The listing builds one solid part. Answer for the finished solid, in the listing's coordinates (mm). A direction names the side the tool comes from. Round coordinates to 2 decimals unless told otherwise and drop trailing zeros. Loops run counter-clockwise (first coordinate to the right, second up) from the corner with the lowest first, then second, coordinate; pieces in that order, holes last. Notation, with made-up numbers: (51, 19) -> (94, 19) arc R14 ccw to (94, 34) -> close; hole circle Ø5 at (-4, 55.5). An arc over 180 degrees is marked (long way). Write each question's results on one line, items separated by ' | '. Start each with the question number.
(1) For faces 5 (the face through (24.599, 16.868, -11.668)), 6 (the face through (22.67, 7.94, -7.07)), 7 (the face through (17.455, 12, -49)), 8 (the face through (18, 18.622, -43)), determine the directions among +Z, -Z, +X, -X, +Y, -Y from which every point of the face is accessible in a straight line to the end or side of a thin tool.
(2) The part is cut by section B-B (y = 4.5). Determine the outline of the cut face in (x, z).
(3) The part is cut by section C-C (x = 15). Determine the outline of the cut face in (y, z), plus the area to 3 significant figures.
(4) Straight lines are drawn through the part: probe 1 along Z at (x, y) = (11.75, 11.5); probe 2 along Y at (x, z) = (18.25, -6). For each, find the intervals that lie inside material, in ascending order.
(5) Determine the mould class of faces 1 (the face through (11.35, 18.05, -42.93)), 2 (the face through (18.144, 12.138, -10.497)), 3 (the face through (18, 0.622, -43)), 4 (the face through (19.226, 12.217, -5.07)) for opening direction Y: released by +Y, released by -Y, zero draft, split by the parting line, or undercut.
(6) The part is cut by section A-A (z = -45). Determine the outline of the cut face in (x, y), plus the area to 3 significant figures.
(7) The part is cut by section D-D (y = 7.5). Determine the outline of the cut face in (x, z).
(8) Flat-ended cylindrical pins translate along their axes: pin 1 (1.6 mm diameter, centred on y = 12, z = -48.5, fed in from +X); pin 2 (1.8 mm diameter, centred on x = 18.25, y = 12, fed in from +Z); pin 3 (3 mm diameter, centred on x = 18.5, z = -45.5, fed in from +Y); pin 4 (5 mm diameter, centred on x = 20, y = 15, fed in from +Z). Find the tip coordinate at first contact, or state that the pin passes through.
Autodesk Inventor part; units mm, degrees
ref_plane "YZ Plane" through (0, 0, 0) normal (1, 0, 0) x (0, 1, 0)
ref_plane "XZ Plane" through (0, 0, 0) normal (0, 1, 0) x (-1, 0, 0)
ref_plane "XY Plane" through (0, 0, 0) normal (0, 0, 1) x (1, 0, 0)
sketch "Sketch1" plane through (0, 0, 0) normal (0, 0, 1) x (1, 0, 0)
  arc A0 (10.5041, 10) -> (25.996, 10) centre (18.25, 12) ccw
  circle A1 centre (18.25, 12) radius 8
  point P0 (0, 0)
extrude "Extrusion1" add sketch "Sketch1" against normal blind 4.8
sketch "Sketch2" plane through (18.25, 12, -4.8) normal (0, 0, -1) x (-1, 0, 0)
  circle A0 centre (0, 0) radius 8
  circle A1 centre (0, 0) radius 6
  point P0 (18.25, -12)
  dimension "d2" = 12
extrude "Extrusion2" add sketch "Sketch2" along normal blind 4.6 contours A1
sketch "Sketch3" plane through (18.25, 12, -9.4) normal (0, 0, -1) x (-1, 0, 0)
  circle A0 centre (0, 0) radius 6
  circle A1 centre (0, 0) radius 8
  point P0 (18.25, -12)
extrude "Extrusion3" add sketch "Sketch3" along normal blind 4.6 contours A0 | A1
sketch "Sketch4" plane through (18.25, 12, -14) normal (0, 0, -1) x (-1, 0, 0)
  circle A0 centre (0, 0) radius 8
  circle A1 centre (0, 0) radius 5
  point P0 (18.25, -12)
  dimension "d7" = 10
extrude "Extrusion4" add sketch "Sketch4" along normal blind 24 contours A1
thread "Thread1"
sketch "Sketch5" plane through (18.25, 12, -38) normal (0, 0, -1) x (-1, 0, 0)
  line L0 (-5.5007, -11.3783) -> (5.4993, -11.3783)
  line L1 (7.4993, -9.3783) -> (7.4993, 4.6217)
  line L2 (5.4993, 6.6217) -> (-5.5007, 6.6217)
  line L3 (-7.5007, 4.6217) -> (-7.5007, -9.3783)
  line L4 (-7.5007, -11.3783) -> (7.4993, 6.6217) construction
  line L5 (7.4993, -11.3783) -> (-7.5007, 6.6217) construction
  arc A0 (7.4993, 4.6217) -> (5.4993, 6.6217) centre (5.4993, 4.6217) ccw
  arc A1 (-5.5007, 6.6217) -> (-7.5007, 4.6217) centre (-5.5007, 4.6217) ccw
  arc A2 (-7.5007, -9.3783) -> (-5.5007, -11.3783) centre (-5.5007, -9.3783) ccw
  arc A3 (5.4993, -11.3783) -> (7.4993, -9.3783) centre (5.4993, -9.3783) ccw
  point P0 (18.25, -12)
  point P1 (-0.0007, -2.3783)
  dimension "d12" = 15
  dimension "d13" = 18
  dimension "d14" = 2
extrude "Extrusion5" add sketch "Sketch5" along normal blind 10
sketch "Sketch6" plane through (18.25, 12, -48) normal (0, 0, -1) x (-1, 0, 0)
  circle A0 centre (0, 0) radius 5
  circle A1 centre (0, 0) radius 1.15
  point P0 (18.25, -12)
  dimension "d17" = 2.3
ref_plane "Work Plane1" through (12.7508, 11.9997, -38) normal (0, 1, 0) x (1, 0, 0)
sketch "Sketch7" plane through (12.7508, 11.9997, -38) normal (0, 1, 0) x (1, 0, 0)
  line L0 (6.6493, 10) -> (4.3493, 10)
  line L1 (5.4993, 10) -> (5.4993, 14.106)
  line L2 (5.3539, 14.106) -> (4.3493, 10)
  line L3 (5.4993, 14.106) -> (5.3539, 14.106)
  line L4 (5.4993, 14.106) -> (5.6446, 14.106) construction
  line L5 (5.4993, 10) -> (4.3493, 10)
  line L6 (4.3493, 10) -> (5.3539, 14.106)
  point P0 (-12.7508, -38)
  dimension "d20" = 180
revolve "Revolution1" add sketch "Sketch7" angle 360 about axis through (18.25, 11.9997, -48) along (0, 0, -1)
sketch "Sketch8" plane through (18.25, 11.9997, -52.106) normal (0, 0, -1) x (-1, 0, 0)
  circle A0 centre (0, 0) radius 0.1454
  circle A1 centre (0, 0) radius 0.1
  point P0 (18.25, -11.9997)
  dimension "d22" = 0.2
extrude "Extrusion6" cut sketch "Sketch8" against normal up to surface (4.106 mm away) contours A1
sketch "Sketch9" plane through (18.25, 12, -48) normal (0, 0, -1) x (-1, 0, 0)
  line L0 (2.1554, 3.8954) -> (0.7949, 3.8954)
  line L1 (0.7949, 3.8954) -> (0.7949, -1.2159)
  line L2 (0.7949, -1.2159) -> (2.1554, -1.2159)
  line L3 (2.1554, -1.2159) -> (2.1554, 3.8954)
  line L4 (2.1554, 3.8954) -> (0.7949, -1.2159) construction
  line L5 (0.7949, 3.8954) -> (2.1554, -1.2159) construction
  line L6 (-2.1285, 4.9618) -> (-0.8047, 4.9618)
  line L7 (-0.8047, 4.9618) -> (-0.8047, -1.2159)
  line L8 (-0.8047, -1.2159) -> (-2.1285, -1.2159)
  line L9 (-2.1285, -1.2159) -> (-2.1285, 4.9618)
  line L10 (-2.1285, 4.9618) -> (-0.8047, -1.2159) construction
  line L11 (-0.8047, 4.9618) -> (-2.1285, -1.2159) construction
  point P0 (18.25, -12)
  point P1 (1.4752, 1.3398)
  point P2 (-1.4666, 1.873)
extrude "Extrusion7" cut sketch "Sketch9" along normal blind 10
sketch "Sketch10" plane through (18.25, 12, 0) normal (0, 0, 1) x (1, 0, 0)
  circle A0 centre (0, 0) radius 8
  point P0 (-18.25, -12)
  point P1 (0.8047, 0.8213)
hole "Hole1" at (18.25, 12, 0) direction (0, 0, -1) diameter 2 depth 10 tip angle 118
properties part number "Hotend Mock Up"
Checked values:
1) face 5: +Z | face 6: none | face 7: -Z, -X, +Y, -Y | face 8: -Z, +X, -X, +Y
2) outline: (10.75, -48) -> (25.75, -48) -> (25.75, -38) -> (10.75, -38) -> close; (15.47, -14) -> (21.03, -14) -> (21.03, -9.4) -> (15.47, -9.4) -> close; (15.47, -4.8) -> (21.03, -4.8) -> (21.03, 0) -> (15.47, 0) -> close
3) outline: (0.62, -48) -> (18.62, -48) -> (18.62, -38) -> (15.8, -38) -> (15.8, -14) -> (19.31, -14) -> (19.31, -9.4) -> (17.04, -9.4) -> (17.04, -4.8) -> (19.31, -4.8) -> (19.31, 0) -> (4.69, 0) -> (4.69, -4.8) -> (6.96, -4.8) -> (6.96, -9.4) -> (4.69, -9.4) -> (4.69, -14) -> (8.2, -14) -> (8.2, -38) -> (0.62, -38) -> close | area: 546 mm2
4) probe 1: z = -48 to -38, -14 to -9.4, -4.8 to 0 | probe 2: y = 6 to 11, 13 to 18
5) face 1: released by +Y | face 2: undercut | face 3: released by -Y | face 4: undercut
6) outline: (10.75, 2.62) arc R2 ccw to (12.75, 0.62) -> (23.75, 0.62) arc R2 ccw to (25.75, 2.62) -> (25.75, 16.62) arc R2 ccw to (23.75, 18.62) -> (12.75, 18.62) arc R2 ccw to (10.75, 16.62) -> close | area: 267 mm2
7) outline: (10.75, -48) -> (25.75, -48) -> (25.75, -38) -> (20.43, -38) -> (20.43, -14) -> (24.86, -14) -> (24.86, -9.4) -> (22.22, -9.4) -> (22.22, -4.8) -> (24.86, -4.8) -> (24.86, 0) -> (11.64, 0) -> (11.64, -4.8) -> (14.28, -4.8) -> (14.28, -9.4) -> (11.64, -9.4) -> (11.64, -14) -> (16.07, -14) -> (16.07, -38) -> (10.75, -38) -> close
8) pin 1: stops at x = 25.75 | pin 2: stops at z = -10.06 | pin 3: stops at y = 18.62 | pin 4: stops at z = 0
